Can you work these out from the model? Positions are in its coordinate system, mm. Face numbers are marked on the shaded views. A direction names the side the tool comes from. Round coordinates to 2 decimals unless told otherwise and drop trailing zeros. Loops run counter-clockwise (first coordinate to the right, second up) from the corner with the lowest first, then second, coordinate; pieces in that order, holes last. Notation, with made-up numbers: (0, -16) -> (20, -16) arc R23 cw to (20, 22) -> close; hole circle Ø4 at (-39, 35). An arc over 180 degrees is marked (long way). Write item = value, one per line.
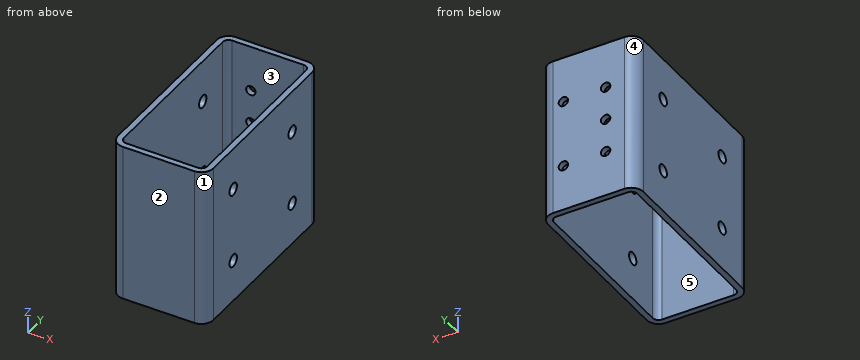
from build123d import *

# Parameters (mm, degrees)
CNC_4X2X0_125_1_DEPTH = 85
SKETCH3_R             = 2.5
CUT_EXTRUDE1_DEPTH    = 10
SKETCH2_R             = 3.3
CUT_EXTRUDE2_DEPTH    = 84.471731742


with BuildPart() as part:
    # Sketch1 → Cnc 4X2X0.125(1) (new body)
    with BuildSketch(Plane.YX.offset(-42.5)):
        with BuildLine():
            Line((44.45, -25.4), (-44.45, -25.4))
            ThreePointArc((-44.45, -25.4), (-48.940128061, -23.540128061), (-50.8, -19.05))
            Line((-50.8, -19.05), (-50.8, 19.05))
            ThreePointArc((-50.8, 19.05), (-48.940128061, 23.540128061), (-44.45, 25.4))
            Line((-44.45, 25.4), (44.45, 25.4))
            ThreePointArc((44.45, 25.4), (48.940128061, 23.540128061), (50.8, 19.05))
            Line((50.8, 19.05), (50.8, -19.05))
            ThreePointArc((50.8, -19.05), (48.940128061, -23.540128061), (44.45, -25.4))
        make_face()
        with BuildLine():
            Line((44.45, 22.225), (-44.45, 22.225))
            ThreePointArc((-44.45, 22.225), (-46.69506403, 21.29506403), (-47.625, 19.05))
            Line((-47.625, 19.05), (-47.625, -19.05))
            ThreePointArc((-47.625, -19.05), (-46.69506403, -21.29506403), (-44.45, -22.225))
            Line((-44.45, -22.225), (44.45, -22.225))
            ThreePointArc((44.45, -22.225), (46.69506403, -21.29506403), (47.625, -19.05))
            Line((47.625, -19.05), (47.625, 19.05))
            ThreePointArc((47.625, 19.05), (46.69506403, 21.29506403), (44.45, 22.225))
        make_face(mode=Mode.SUBTRACT)
    extrude(amount=CNC_4X2X0_125_1_DEPTH)

    # Sketch3 → Cut-Extrude1 (cut)
    with BuildSketch(Plane(origin=(0, 50.8, 0), x_dir=(1, 0, 0), z_dir=(0, 1, 0))):
        with Locations(Location((-9.1, 18, 0), (0, 0, 180))):
            Circle(SKETCH3_R)
        with Locations(Location((-9.1, 0, 0), (0, 0, 180))):
            Circle(SKETCH3_R)
        with Locations(Location((-9.1, -18, 0), (0, 0, 180))):
            Circle(SKETCH3_R)
        with Locations(Location((13.4, 18, 0), (0, 0, 180))):
            Circle(SKETCH3_R)
        with Locations(Location((13.4, -18, 0), (0, 0, 180))):
            Circle(SKETCH3_R)
    extrude(amount=-CUT_EXTRUDE1_DEPTH, mode=Mode.SUBTRACT)

    # Sketch2 → Cut-Extrude2 (cut, through all)
    with BuildSketch(Plane(origin=(25.4, 0, 0), x_dir=(0, 0, -1), z_dir=(1, 0, 0))):
        with Locations(Location((-20, 26.5, 0), (0, 0, 90))):
            Circle(SKETCH2_R)
        with Locations(Location((20, 26.5, 0), (0, 0, 90))):
            Circle(SKETCH2_R)
        with Locations(Location((20, -26.5, 0), (0, 0, 90))):
            Circle(SKETCH2_R)
        with Locations(Location((-20, -26.5, 0), (0, 0, 90))):
            Circle(SKETCH2_R)
    extrude(amount=-CUT_EXTRUDE2_DEPTH, mode=Mode.SUBTRACT)


solid = part.part
1. For the marked faces 4 and 5, which set-ups out of +Z, -Z, +X, -X, +Y, -Y let a thin tool reach every point of the face, with its end or its side?
Entries:
face_4 = +Z, -Z, -X, +Y
face_5 = +Z, -Z
2. Suppose I cut it at C-C, the plane x = -9.1. List the corners of the cut face in (y, z) for me (3 decimals), and give its area (3 significant figures).
Entries:
outline = (-50.8, -42.5) -> (-47.625, -42.5) -> (-47.625, 42.5) -> (-50.8, 42.5) -> close; (47.625, -42.5) -> (50.8, -42.5) -> (50.8, -20.5) -> (47.625, -20.5) -> close; (47.625, -15.5) -> (50.8, -15.5) -> (50.8, -2.5) -> (47.625, -2.5) -> close; (47.625, 2.5) -> (50.8, 2.5) -> (50.8, 15.5) -> (47.625, 15.5) -> close; (47.625, 20.5) -> (50.8, 20.5) -> (50.8, 42.5) -> (47.625, 42.5) -> close
area = 492 mm²
3. I need wall thicknesses on line 1 (Z direction, x = -22.9, y = -26.5); line 2 (Z direction, x = -9.1, y = 49.25); line 3 (X direction, y = 27, z = -11) (3 decimals). Which ranges of each line are inside material? Lowest first, please. Write a range as [from, to].
Entries:
line_1 = [-42.5, -23.3], [-16.7, 16.7], [23.3, 42.5]
line_2 = [-42.5, -20.5], [-15.5, -2.5], [2.5, 15.5], [20.5, 42.5]
line_3 = [-25.4, -22.225], [22.225, 25.4]
4. We'd pull the mould along X, two halves only. Please class the marked faces 1, 2 and 3: released by +X, released by -X, zero draft, split by the parting line, or undercut.
Entries:
face_1 = released by +X
face_2 = zero draft
face_3 = undercut
5. Suppose I cut it at A-A, the plane y = -26.5. List the corners of the cut face in (x, z) for me (3 decimals).
Entries:
outline = (-25.4, -42.5) -> (-22.225, -42.5) -> (-22.225, -23.3) -> (-25.4, -23.3) -> close; (-25.4, -16.7) -> (-22.225, -16.7) -> (-22.225, 16.7) -> (-25.4, 16.7) -> close; (-25.4, 23.3) -> (-22.225, 23.3) -> (-22.225, 42.5) -> (-25.4, 42.5) -> close; (22.225, -42.5) -> (25.4, -42.5) -> (25.4, -23.3) -> (22.225, -23.3) -> close; (22.225, -16.7) -> (25.4, -16.7) -> (25.4, 16.7) -> (22.225, 16.7) -> close; (22.225, 23.3) -> (25.4, 23.3) -> (25.4, 42.5) -> (22.225, 42.5) -> close
6. Suppose I cut it at B-B, the plane z = -5. List the corners of the cut face in (x, y) for me (3 decimals), and give its area (3 significant figures).
Entries:
outline = (-25.4, -44.45) arc R6.35 ccw to (-19.05, -50.8) -> (19.05, -50.8) arc R6.35 ccw to (25.4, -44.45) -> (25.4, 44.45) arc R6.35 ccw to (19.05, 50.8) -> (-19.05, 50.8) arc R6.35 ccw to (-25.4, 44.45) -> close; hole (-22.225, -44.45) arc R3.175 ccw to (-19.05, -47.625) -> (19.05, -47.625) arc R3.175 ccw to (22.225, -44.45) -> (22.225, 44.45) arc R3.175 ccw to (19.05, 47.625) -> (-19.05, 47.625) arc R3.175 ccw to (-22.225, 44.45) -> close
area = 901 mm²
7. Suppose I cut it at D-D, the plane y = 11. List the corners of the cut face in (x, z) for me (3 decimals), and give its area (3 significant figures).
Entries:
outline = (-25.4, -42.5) -> (-22.225, -42.5) -> (-22.225, 42.5) -> (-25.4, 42.5) -> close; (22.225, -42.5) -> (25.4, -42.5) -> (25.4, 42.5) -> (22.225, 42.5) -> close
area = 540 mm²
8. I'm going to push flat-ended pins straight in: pin 1 (4.5 mm diameter, centred on x = 13.4, z = -18, fed in from +Y) (3 decimals); pin 2 (4 mm diameter, centred on y = -26.5, z = 20, fed in from -X). Where does each tip first touch, or does it pass through?
Entries:
pin_1 = -47.625
pin_2 = through
